```python
from build123d import *

# Parameters (mm, degrees)
F1_DEPTH = 2.3368


with BuildPart() as f1:
    # F0 (on Front) → F1 (new body)
    with BuildSketch(Plane.XZ):
        Polygon((1326.235613, 2.9e-05), (1.3e-05, 2.9e-05), (1.3e-05, -400.811971), (-64.261987, -400.811971), (-64.261987, -666.749971), (1389.888013, -666.749971), (1389.888013, -406.399971), (1326.235613, -406.399971), align=None)
    extrude(amount=F1_DEPTH)


solid = f1.part
```
Geometry check sheet. Reference: the model listing, model coordinates, mm. Give positions to 0.01 mm unless a question says otherwise; leave off trailing zeros. Write each loop counter-clockwise with the first axis right and the second up, starting at its lowest first coordinate (ties: lowest second). Pieces come first, ordered by that corner, then holes.
1) Gauge pin test, flat ends, axial feed: pin 1 (0.7 mm diameter, centred on y = -1, z = -165, fed in from +X); pin 2 (1.2 mm diameter, centred on x = -22.5, y = -1, fed in from +Z); pin 3 (1.2 mm diameter, centred on x = 1371, y = -1.5, fed in from +Z). Record the tip position at first contact, or that the pin passes through.
2) Section check A-A, the plane y = -0.95. Record the boundary of the cut face in (x, z).
3) Section check B-B, the plane z = -181. Record the boundary of the cut face in (x, y).
4) Material ranges on L1, parallel to X at y = -2.1, z = -366, recorded low to high.
Computed:
1. pin 1: stops at x = 1326.24
1. pin 2: stops at z = -400.81
1. pin 3: stops at z = -406.4
2. outline: (-64.26, -666.75) - (1389.89, -666.75) - (1389.89, -406.4) - (1326.24, -406.4) - (1326.24, 0) - (0, 0) - (0, -400.81) - (-64.26, -400.81) - close
3. outline: (0, -2.34) - (1326.24, -2.34) - (1326.24, 0) - (0, 0) - close
4. L1: x = 0 to 1326.24
